from build123d import *

# Parameters (mm, degrees)
PAD_DEPTH    = 25
SKETCH001_R  = 1.1
POCKET_DEPTH = 16.001


with BuildPart() as part:
    # Sketch → Pad (new body)
    with BuildSketch(Plane.XY):
        with BuildLine():
            Line((-15.716234, -3), (-20, -3))
            Line((-20, -3), (-20, 0))
            Line((-20, 0), (-14, 0))
            ThreePointArc((-14, 0), (0, -14), (14, 0))
            Line((14, 0), (20, 0))
            Line((20, 0), (20, -3))
            Line((20, -3), (15.716234, -3))
            ThreePointArc((-15.716234, -3), (0, -16), (15.716234, -3))
        make_face()
    extrude(amount=PAD_DEPTH)

    # Sketch001 → Pocket (cut, through all)
    with BuildSketch(Plane(origin=(0, 0, 0), x_dir=(-1, 0, 0), z_dir=(0, 1, 0))):
        with Locations((-17, 22)):
            Circle(SKETCH001_R)
        with Locations((-17, 12)):
            Circle(SKETCH001_R)
        with Locations((17, 22)):
            Circle(SKETCH001_R)
        with Locations((17, 12)):
            Circle(SKETCH001_R)
    extrude(amount=-POCKET_DEPTH, mode=Mode.SUBTRACT)


solid = part.part
Read the model definition and answer for the solid it produces. Units are mm, in the model's axes. A direction names the side the tool comes from. Round coordinates to 2 decimals unless told otherwise and drop trailing zeros. Order: outer loops, then holes, each group sorted by start corner. A loop starts at its lowest first (then second) coordinate and runs counter-clockwise, first axis right, second up.
1) Flat-ended cylindrical pins translate along their axes: pin 1 (2 mm diameter, centred on x = -9.5, z = 14, fed in from +Y); pin 2 (2 mm diameter, centred on x = -17, z = 22, fed in from +Y); pin 3 (4 mm diameter, centred on y = -10, z = 22, fed in from -X); pin 4 (6 mm diameter, centred on x = -12.5, z = 18, fed in from -Y). Find the tip coordinate at first contact, or state that the pin passes through.
2) For faces 1 (the face through (18.4, -3, 12.3)), 2 (the face through (0, -14, 12)), determine the directions among +Z, -Z, +X, -X, +Y, -Y from which every point of the face is accessible in a straight line to the end or side of a thin tool.
3) The part is cut by section B-B on x = -17. Write down the section's boundary in (y, z), plus the area to 3 significant figures.
4) The mould has two halves that part along Z. Classify faces 3 (the face through (17.87, -1.48, 21.33)), 4 (the face through (0.1, -14.5, 25)), 5 (the face through (-18.3, -3, 12.3)): released by +Z, released by -Z, zero draft, split by the parting line, or undercut.
5) The part is cut by section D-D on y = -1. Write down the section's boundary in (x, z).
6) Straight lines are drawn through the part: L1, parallel to Z at x = -17, y = -1.15; L2, parallel to X at y = -2.25, z = 22.25; L3, parallel to Y at x = 16, z = 7. For each, find the intervals that lie inside material, in ascending order.
7) The part is cut by section A-A on z = 22. Write down the section's boundary in (x, y).
8) The part is cut by section C-C on y = -9.25. Write down the section's boundary in (x, z), plus the area to 3 significant figures.
Resolved:
1. pin 1: stops at y = -9.26
1. pin 2: passes through
1. pin 3: stops at x = -13.86
1. pin 4: stops at y = -12.87
2. face 1: +Z, -Z, +X, -Y
2. face 2: +Z, -Z, +Y
3. outline: (-3, 0) - (0, 0) - (0, 10.9) - (-3, 10.9) - close; (-3, 13.1) - (0, 13.1) - (0, 20.9) - (-3, 20.9) - close; (-3, 23.1) - (0, 23.1) - (0, 25) - (-3, 25) - close
3. area: 61.8 mm2
4. face 3: undercut
4. face 4: released by +Z
4. face 5: zero draft
5. outline: (-20, 0) - (-13.96, 0) - (-13.96, 25) - (-20, 25) - close; (13.96, 0) - (20, 0) - (20, 25) - (13.96, 25) - close; hole circle Ø2.2 at (-17, 12); hole circle Ø2.2 at (-17, 22); hole circle Ø2.2 at (17, 12); hole circle Ø2.2 at (17, 22)
6. L1: z = 0 to 10.9, 13.1 to 20.9, 23.1 to 25
6. L2: x = -20 to -18.07, -15.93 to -13.82, 13.82 to 15.93, 18.07 to 20
6. L3: y = -3 to 0
7. outline: (-20, -3) - (-18.1, -3) - (-18.1, 0) - (-20, 0) - close; (-15.9, -3) - (-15.72, -3) arc R16 ccw to (15.72, -3) - (15.9, -3) - (15.9, 0) - (14, 0) arc R14 cw to (-14, 0) - (-15.9, 0) - close; (18.1, -3) - (20, -3) - (20, 0) - (18.1, 0) - close
8. outline: (-13.06, 0) - (-10.51, 0) - (-10.51, 25) - (-13.06, 25) - close; (10.51, 0) - (13.06, 0) - (13.06, 25) - (10.51, 25) - close
8. area: 127 mm2
